from build123d import *

# Parameters (mm, degrees)
SKETCH_1_W      = 143
SKETCH_1_H      = 8
SKETCH_1_R      = 1.6
EXTRUDE_1_DEPTH = 4
SKETCH_2_W      = 107
SKETCH_2_H      = 2.5
EXTRUDE_2_DEPTH = 21
SKETCH_3_W      = 143
SKETCH_3_H      = 12
SKETCH_3_R      = 1.6
EXTRUDE_4_DEPTH = 4
FILLET_1_R      = 2


with BuildPart() as part:
    # 草图1 → 凸台-拉伸1 (new body)
    with BuildSketch(Plane.XY):
        Rectangle(SKETCH_1_W, SKETCH_1_H)
        with Locations((-67.5, 0)):
            Circle(SKETCH_1_R, mode=Mode.SUBTRACT)
        with Locations((-57.5, 0)):
            Circle(SKETCH_1_R, mode=Mode.SUBTRACT)
        with Locations((57.5, 0)):
            Circle(SKETCH_1_R, mode=Mode.SUBTRACT)
        with Locations((67.5, 0)):
            Circle(SKETCH_1_R, mode=Mode.SUBTRACT)
    extrude(amount=EXTRUDE_1_DEPTH)

    # 草图2 → 凸台-拉伸2 (add)
    with BuildSketch(Plane.XY.offset(4)):
        with Locations((0, 2.75)):
            Rectangle(SKETCH_2_W, SKETCH_2_H)
    extrude(amount=EXTRUDE_2_DEPTH)

    # 草图3 → 凸台-拉伸4 (add)
    with BuildSketch(Plane.XY.offset(25)):
        with Locations((0, 7.5)):
            Rectangle(SKETCH_3_W, SKETCH_3_H)
        with Locations((67.5, 7.5)):
            Circle(SKETCH_3_R, mode=Mode.SUBTRACT)
        with Locations((57.5, 7.5)):
            Circle(SKETCH_3_R, mode=Mode.SUBTRACT)
        with Locations((-67.5, 7.5)):
            Circle(SKETCH_3_R, mode=Mode.SUBTRACT)
        with Locations((-57.5, 7.5)):
            Circle(SKETCH_3_R, mode=Mode.SUBTRACT)
    extrude(amount=EXTRUDE_4_DEPTH)

    # 圆角1
    fillet_1_edges = [part.edges().sort_by_distance(p)[0] for p in [
        (53.5, 2.75, 25),
        (-53.5, 2.75, 4),
        (-53.5, 2.75, 25),
        (53.5, 2.75, 4),
        (-71.5, 13.5, 27),
        (-71.5, 1.5, 27),
        (71.5, 1.5, 27),
        (71.5, 13.5, 27),
        (71.5, -4, 2),
        (-71.5, -4, 2),
        (-71.5, 4, 2),
        (71.5, 4, 2),
    ]]
    fillet(fillet_1_edges, radius=FILLET_1_R)


solid = part.part
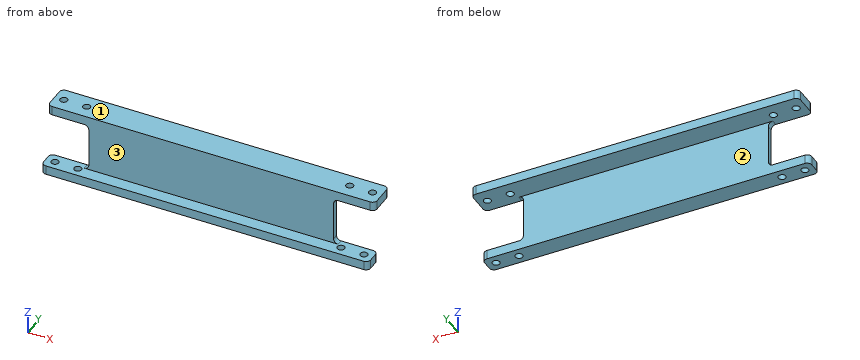
Input: part model. Units: mm. Frame: model coordinates. Face numbers are marked on the shaded views. A direction names the side the tool comes from. Round coordinates to 2 decimals unless told otherwise and drop trailing zeros. Write each loop counter-clockwise with the first axis right and the second up, starting at its lowest first coordinate (ties: lowest second). Pieces come first, ordered by that corner, then holes.
1) Contact query for flat-ended pins moving along their axis: P1, Ø2, axis at x = 29.5, z = 23, coming from the +Y side; P2, Ø7.5, axis at x = 29, z = 14, coming from the -Y side; P3, Ø3, axis at y = 2.5, z = 13.5, coming from the -X side. Output: stop coordinate, or through.
2) Cut plane B-B (x = -67.5). Return the cut outline in (y, z).
3) Cut plane D-D (z = 26.5). Return the cut outline in (x, y), then the cut area to 3 significant figures.
4) Cut plane C-C (x = -50). Return the cut outline in (y, z).
5) Cut plane A-A (y = 0). Return the cut outline in (x, z), then the cut area to 3 significant figures.
6) Ray query, L1, parallel to Y at x = -67.5, z = 25.85; L2, parallel to Y at x = -67.5, z = 1.95; L3, parallel to Z at x = -63.5, y = 9.25. Return the intervals inside material, ascending.
7) Reachability of the marked faces 1, 2 and 3 from +Z, -Z, +X, -X, +Y, -Y: full face, straight path, thin tool, end or side. Return the list, or none.
Geometry says:
1. P1: stops at y = 4
1. P2: stops at y = 1.5
1. P3: stops at x = -53.5
2. outline: (-4, 0) - (-1.6, 0) - (-1.6, 4) - (-4, 4) - close; (1.5, 25) - (5.9, 25) - (5.9, 29) - (1.5, 29) - close; (1.6, 0) - (4, 0) - (4, 4) - (1.6, 4) - close; (9.1, 25) - (13.5, 25) - (13.5, 29) - (9.1, 29) - close
3. outline: (-71.5, 3.5) arc R2 ccw to (-69.5, 1.5) - (69.5, 1.5) arc R2 ccw to (71.5, 3.5) - (71.5, 11.5) arc R2 ccw to (69.5, 13.5) - (-69.5, 13.5) arc R2 ccw to (-71.5, 11.5) - close; hole circle Ø3.2 at (-67.5, 7.5); hole circle Ø3.2 at (-57.5, 7.5); hole circle Ø3.2 at (57.5, 7.5); hole circle Ø3.2 at (67.5, 7.5)
3. area: 1,680 mm2
4. outline: (-4, 0) - (4, 0) - (4, 25) - (13.5, 25) - (13.5, 29) - (1.5, 29) - (1.5, 4) - (-4, 4) - close
5. outline: (-71.5, 0) - (-69.1, 0) - (-69.1, 4) - (-71.5, 4) - close; (-65.9, 0) - (-59.1, 0) - (-59.1, 4) - (-65.9, 4) - close; (-55.9, 0) - (55.9, 0) - (55.9, 4) - (-55.9, 4) - close; (59.1, 0) - (65.9, 0) - (65.9, 4) - (59.1, 4) - close; (69.1, 0) - (71.5, 0) - (71.5, 4) - (69.1, 4) - close
5. area: 521 mm2
6. L1: y = 1.5 to 5.9, 9.1 to 13.5
6. L2: y = -4 to -1.6, 1.6 to 4
6. L3: z = 25 to 29
7. face 1: +Z, +X, -X, +Y, -Y
7. face 2: -Z, +X, -X, +Y
7. face 3: +Z, +X, -X, -Y
